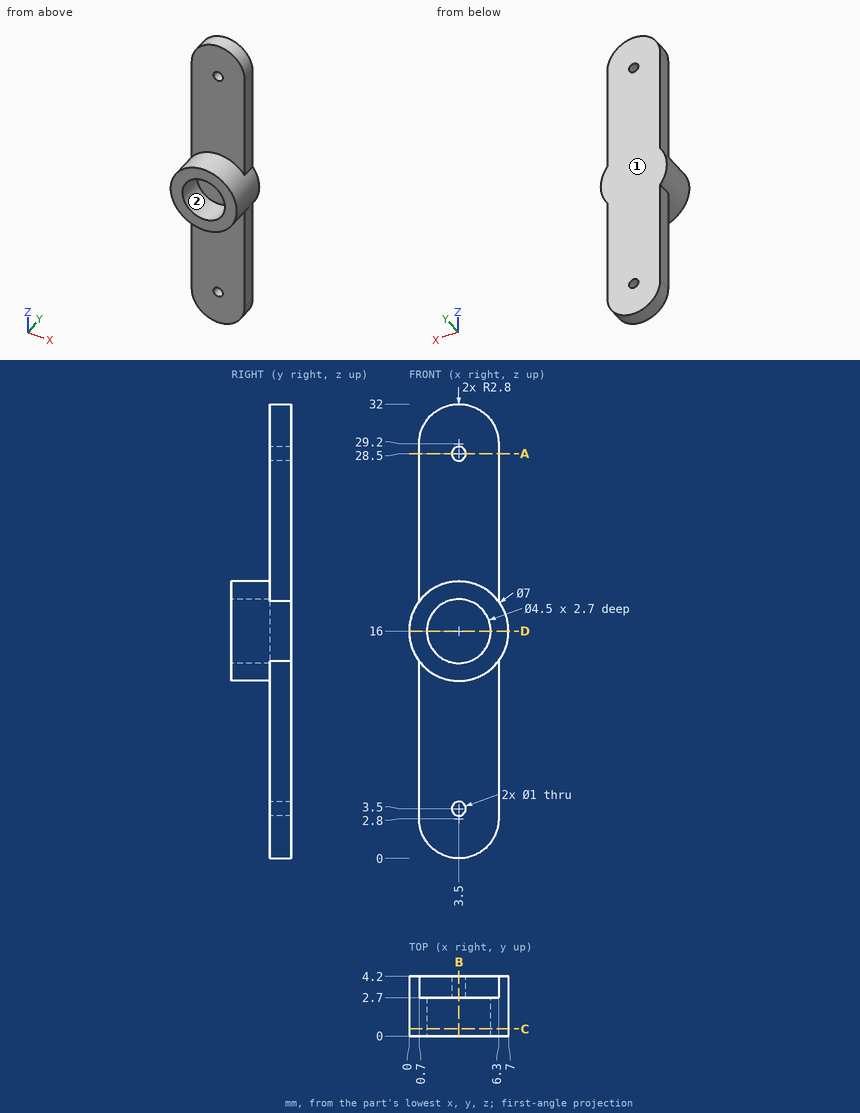
Job drawing, mm, ordinate dimensions from the low corner. One solid piece. A direction names the side the tool comes from. Coordinates: 2 decimals unless noted, no trailing zeros. Write each loop counter-clockwise with the first axis right and the second up, starting at its lowest first coordinate (ties: lowest second). Pieces come first, ordered by that corner, then holes. Notation, with made-up numbers: (9.5, 11) -> (27.5, 11) arc R27 ccw to (27.5, 46) -> close; hole circle Ø9 at (81, 81.25). An arc over 180 degrees is marked (long way). Use CSV: the item, a comma, the result in double quotes. Start each with the question number.
Item 1: Band-saw the part on D-D, the plane z = 16. Write the cut outline in (x, y).
Item 2: Band-saw the part on B-B, the plane x = 3.5. Write the cut outline in (y, z), plus the area to 4 significant figures.
Item 3: Tool access for the marked faces 1 and 2: list every direction of +Z, -Z, +X, -X, +Y, -Y with a clear straight run to the whole face (end or side of a thin tool).
Item 4: Wall check: probe 1 along Z at (x, y) = (3.5, 3.7); probe 2 along Z at (x, y) = (3.5, 2.35); probe 3 along Y at (x, z) = (3, 5). Give the ranges that are in metal, low to high.
Item 5: Band-saw the part on C-C, the plane y = 0.5. Write the cut outline in (x, z).
Item 6: Drop flat-ended pins along their axis: P1, Ø1.5, axis at x = 6, z = 10, coming from the -Y side; P2, Ø1, axis at y = 4, z = 9.5, coming from the -X side; P3, Ø0.8, axis at y = 3.5, z = 24, coming from the +X side. Give the stop position or say it passes through.
Item 7: Band-saw the part on A-A, the plane z = 28.5. Write the cut outline in (x, y), plus the area to 3 significant figures.
Response values:
1,outline,"(0, 0) -> (1.25, 0) -> (1.25, 2.7) -> (5.75, 2.7) -> (5.75, 0) -> (7, 0) -> (7, 4.2) -> (0, 4.2) -> close"
2,outline,"(0, 12.5) -> (2.7, 12.5) -> (2.7, 4) -> (4.2, 4) -> (4.2, 28) -> (2.7, 28) -> (2.7, 19.5) -> (0, 19.5) -> (0, 18.25) -> (2.7, 18.25) -> (2.7, 13.75) -> (0, 13.75) -> close; (2.7, 0) -> (4.2, 0) -> (4.2, 3) -> (2.7, 3) -> close; (2.7, 29) -> (4.2, 29) -> (4.2, 32) -> (2.7, 32) -> close"
2,area,"51.75 mm2"
3,face 1,"+Z, -Z, +X, -X, +Y"
3,face 2,"-Y"
4,probe 1,"z = 0 to 3, 4 to 28, 29 to 32"
4,probe 2,"z = 12.5 to 13.75, 18.25 to 19.5"
4,probe 3,"y = 2.7 to 4.2"
5,outline,"circle Ø7 at (3.5, 16); hole circle Ø4.5 at (3.5, 16)"
6,P1,"stops at y = 2.7"
6,P2,"stops at x = 0.7"
6,P3,"stops at x = 6.3"
7,outline,"(0.7, 2.7) -> (3, 2.7) -> (3, 4.2) -> (0.7, 4.2) -> close; (4, 2.7) -> (6.3, 2.7) -> (6.3, 4.2) -> (4, 4.2) -> close"
7,area,"6.90 mm2"
